Model file for the job. Use its own axes, mm. Face numbers are marked on the shaded views. Give positions to 0.01 mm unless a question says otherwise; leave off trailing zeros. Write each loop counter-clockwise with the first axis right and the second up, starting at its lowest first coordinate (ties: lowest second). Pieces come first, ordered by that corner, then holes. Notation, with made-up numbers: (3.5, 2.5) - (16.5, 2.5) arc R22 cw to (16.5, 38.5) - close; hole circle Ø8 at (55, 31). An arc over 180 degrees is marked (long way). One line per item, written item: value. Start each with the question number.
(1) Probe L1, parallel to Y at x = 0, z = 0.3; L2, parallel to Z at x = 5.5, y = -0.5. List the from-to ranges inside material, lowest first.
(2) Mould opens along Y. For the marked faces 1 and 2 say: pulls with the +Y half, pulls with the -Y half, needs draft (parallel to the pull), parting line crosses it, or undercut.
(3) Cut at A-A, the plane x = 0. List the corners of the cut face in (y, z).
from build123d import *

# Parameters (mm, degrees)
SKETCH1_W           = 400
SKETCH1_H           = 100
BOSS_EXTRUDE1_DEPTH = 10
SKETCH2_R           = 20
CUT_EXTRUDE1_DEPTH  = 0.5


with BuildPart() as part:
    # Sketch1 → Boss-Extrude1 (new body)
    with BuildSketch(Plane.XY):
        Rectangle(SKETCH1_W, SKETCH1_H)
    extrude(amount=BOSS_EXTRUDE1_DEPTH)

    # Sketch2 → Cut-Extrude1 (cut)
    with BuildSketch(Plane(origin=(0, 0, 0), x_dir=(-1, 0, 0), z_dir=(0, 0, -1))):
        Circle(SKETCH2_R)
    extrude(amount=-CUT_EXTRUDE1_DEPTH, mode=Mode.SUBTRACT)


solid = part.part
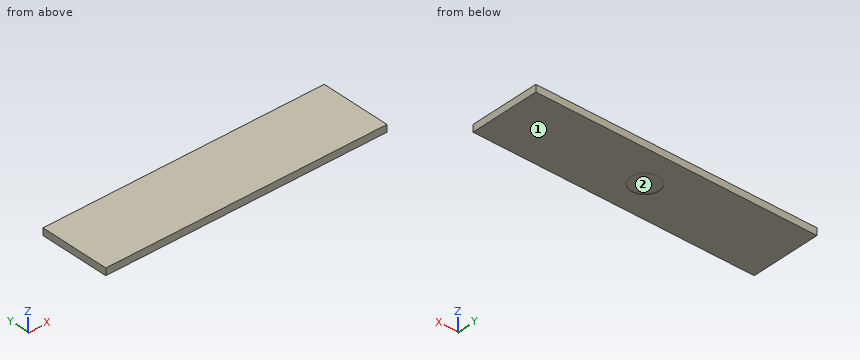
Answers follow:
1. L1: y = -50 to -20, 20 to 50
1. L2: z = 0.5 to 10
2. face 1: needs draft
2. face 2: undercut
3. outline: (-50, 0) - (-20, 0) - (-20, 0.5) - (20, 0.5) - (20, 0) - (50, 0) - (50, 10) - (-50, 10) - close
